For this review, take the finished solid that the model builds, in its own axes (mm). Face numbers are marked on the shaded views. Coordinates: 2 decimals unless noted, no trailing zeros. Write each loop counter-clockwise with the first axis right and the second up, starting at its lowest first coordinate (ties: lowest second). Pieces come first, ordered by that corner, then holes. Notation, with made-up numbers: (-32, 8.5) - (27, 8.5) arc R22 cw to (27, 28.5) - close; hole circle Ø4 at (32, 79.5). An arc over 180 degrees is marked (long way). Use one line per item in the form item = value. Start each with the question number.
1) We need section C-C (y = 11.5). Give the boundary of the cut face in (x, z).
2) We need section A-A (z = 0). Give the boundary of the cut face in (x, y), plus the area to 3 significant figures.
3) Insertion check: P1, Ø10, axis at y = 34.5, z = -9, coming from the +X side; P2, Ø4, axis at y = 37.5, z = -64, coming from the +X side; P3, Ø10, axis at y = 45.5, z = -101, coming from the +X side. Each pin has a flat end and moves straight along its axis. Give the tip position at first contact, or say it passes through.
4) Mouldability with a two-part tool opening along X and no side actions: class the marked faces 1, 2, 3 and 4 as pulls with the +X half, pulls with the -X half, needs draft (parallel to the pull), parting line crosses it, or undercut.
5) We need section D-D (x = 304.5). Give the boundary of the cut face in (y, z).
6) We need section B-B (x = -353). Give the boundary of the cut face in (y, z), plus the area to 3 significant figures.
7) For L1, parallel to X at y = 31.5, z = 3.5; L2, parallel to Z at x = 317, y = 30; L3, parallel to X at y = 42, z = -38, list the stretches that pass through material, from the lowest coordinate up. Write a range as from..to.
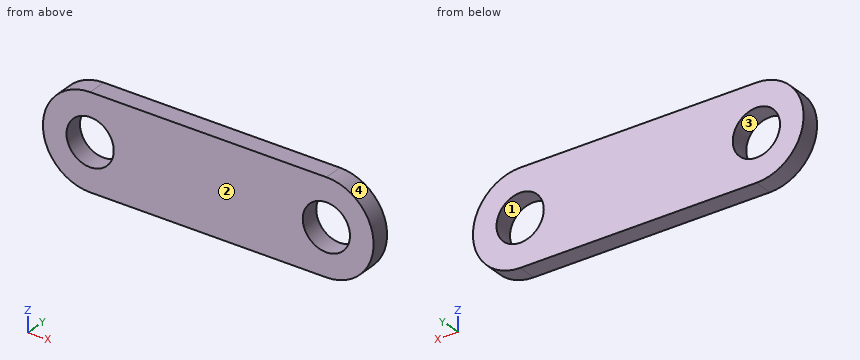
Autodesk Inventor part; units mm, degrees
ref_plane "YZ Plane" through (0, 0, 0) normal (1, 0, 0) x (0, 1, 0)
ref_plane "XZ Plane" through (0, 0, 0) normal (0, 1, 0) x (-1, 0, 0)
ref_plane "XY Plane" through (0, 0, 0) normal (0, 0, 1) x (1, 0, 0)
sketch "Sketch1" plane through (0, 0, 0) normal (0, 1, 0) x (-1, 0, 0)
  line L0 (-317.5, 127) -> (317.5, 127)
  line L1 (317.5, 127) -> (317.5, -127) construction
  line L2 (317.5, -127) -> (-317.5, -127)
  line L3 (-317.5, -127) -> (-317.5, 127) construction
  line L4 (-317.5, 127) -> (317.5, -127) construction
  line L5 (317.5, 127) -> (-317.5, -127) construction
  arc A0 (317.5, -127) -> (317.5, 127) centre (317.5, 0) ccw
  arc A1 (-317.5, 127) -> (-317.5, -127) centre (-317.5, 0) ccw
  circle A2 centre (317.5, 0) radius 63.5
  circle A3 centre (-317.5, 0) radius 63.5
  point P0 (0, 0)
  dimension "d0" = 635
  dimension "d1" = 254
  dimension "d2" = 127
  dimension "d3" = 127
extrude "Extrusion1" add sketch "Sketch1" along normal blind 50.8
properties part number "Input"
Determined:
q1.outline = (-317.5, -127) - (317.5, -127) arc R127 ccw to (317.5, 127) - (-317.5, 127) arc R127 ccw to start; hole circle Ø127 at (-317.5, 0); hole circle Ø127 at (317.5, 0)
q2.outline = (-444.5, 0) - (-381, 0) - (-381, 50.8) - (-444.5, 50.8) - close; (-254, 0) - (254, 0) - (254, 50.8) - (-254, 50.8) - close; (381, 0) - (444.5, 0) - (444.5, 50.8) - (381, 50.8) - close
q2.area = 32,300 mm²
q3.P1 = 444.44
q3.P2 = 428.34
q3.P3 = 400.64
q4.face_1 = undercut
q4.face_2 = needs draft
q4.face_3 = undercut
q4.face_4 = pulls with the +X half
q5.outline = (0, -127) - (50.8, -127) - (50.8, -62.16) - (0, -62.16) - close; (0, 62.16) - (50.8, 62.16) - (50.8, 127) - (0, 127) - close
q6.outline = (0, -121.94) - (50.8, -121.94) - (50.8, -52.65) - (0, -52.65) - close; (0, 52.65) - (50.8, 52.65) - (50.8, 121.94) - (0, 121.94) - close
q6.area = 7,040 mm²
q7.L1 = -444.45..-380.9, -254.1..254.1, 380.9..444.45
q7.L2 = -127..-63.5, 63.5..127
q7.L3 = -438.68..-368.37, -266.63..266.63, 368.37..438.68
